Work out the finished part from the listing and answer in its coordinate system (mm). A direction names the side the tool comes from. Round coordinates to 2 decimals unless told otherwise and drop trailing zeros. Order: outer loops, then holes, each group sorted by start corner. A loop starts at its lowest first (then second) coordinate and runs counter-clockwise, first axis right, second up. Notation, with made-up numbers: (27.5, 14) -> (38.5, 14) arc R26 cw to (38.5, 39) -> close; hole circle Ø9 at (33.5, 19). An arc over 180 degrees is marked (long way). Use a Markdown table: item, result. Add a question column.
Item 1: A cutting plane is placed at C-C, the plane y = 7. Determine the outline of the cut face in (x, z).
Item 2: A cutting plane is placed at B-B, the plane z = -42.25. Determine the outline of the cut face in (x, y).
Item 3: A tool of negligible diameter and unlimited length cuts with its end or side. For faces 4 (the flat face through (35.5, -5, -46)), 5 (the flat face through (64, 0, -59)), 6 (the flat face through (48.733, 0, -46)), 7 (the flat face through (58, 0, -32)), from which of +Z, -Z, +X, -X, +Y, -Y can it reach the whole face along a straight path? Write none if from no direction.
Item 4: A cutting plane is placed at D-D, the plane x = 69. Determine the outline of the cut face in (y, z), plus the area to 3 significant figures.
Item 5: For a pull along Y with two mould halves and no side action, classify faces 1 (the flat face through (58, 0, -60)), 2 (the flat face through (34, -8, -46)), 3 (the flat face through (56, -10, -46)) as +Y half, -Y half, draft (parallel to the pull), parting line (faces both ways), or undercut.
Item 6: A cutting plane is placed at A-A, the plane y = 0. Determine the outline of the cut face in (x, z), plus the area to 3 significant figures.
Item 7: Flat-ended cylindrical pins translate along their axes: P1, Ø1.5, axis at y = 6, z = -44.5, coming from the +X side; P2, Ø5, axis at y = -3, z = -40, coming from the +X side; P3, Ø8, axis at x = 63.5, z = -46.5, coming from the -Y side. Find the tip coordinate at first contact, or state that the pin passes through.
Item 8: Find the intervals of material crossed by L1, parallel to X at y = 8.5, z = -42; L2, parallel to X at y = 1, z = -57.5; L3, parallel to X at y = -5.5, z = -52, in increasing order. Write a range as [from, to].
from build123d import *

# Parameters (mm, degrees)
PAD006_DEPTH            = 28
SKETCH015_W             = 8
SKETCH015_H             = 3
SKETCH015_W_2           = 15
SKETCH015_H_2           = 6
POCKET006_DEPTH         = 28.001
SKETCH016_W             = 20
SKETCH016_H             = 2.5
SKETCH016_W_2           = 18
SKETCH016_H_2           = 3
POCKET007_DEPTH         = 27.001
BODY005_PLACEMENT_ANGLE = 90


with BuildPart() as part:
    # Sketch014 → Pad006 (new body)
    with BuildSketch(Plane.XY):
        with BuildLine():
            Line((-3, -3), (-8, -3))
            Line((-8, -3), (-8, 0))
            Line((-8, 0), (8, 0))
            Line((8, 0), (8, -3))
            Line((8, -3), (3, -3))
            Line((3, -3), (3, -8))
            ThreePointArc((-3, -8), (0, -41.733201), (3, -8))
            Line((-3, -3), (-3, -8))
        make_face()
    extrude(amount=PAD006_DEPTH)

    # Sketch015 (on Face9 of Pad006) → Pocket006 (cut, through all)
    with BuildSketch(Plane(origin=(0, 0, 0), x_dir=(1, 0, 0), z_dir=(0, 0, -1))):
        with Locations((0, 29.733201)):
            Rectangle(SKETCH015_W, SKETCH015_H)
        with Locations((0, 19.233201)):
            Rectangle(SKETCH015_W_2, SKETCH015_H_2)
    extrude(amount=-POCKET006_DEPTH, mode=Mode.SUBTRACT)

    # Sketch016 (on Face4 of Pocket006) → Pocket007 (cut, through all)
    with BuildSketch(Plane(origin=(0, 0, 1), x_dir=(1, 0, 0), z_dir=(0, 0, -1))):
        with Locations((0, 23.483201)):
            Rectangle(SKETCH016_W, SKETCH016_H)
        with Locations((0, 30.933201)):
            Rectangle(SKETCH016_W_2, SKETCH016_H_2)
    extrude(amount=-POCKET007_DEPTH, mode=Mode.SUBTRACT)


with BuildPart() as part_1:
    # Body005 placement: moved
    add(part.part.moved(Location((32.5, 0, -60))).rotate(Axis((32.5, 0, -60), (0, 0, 1)), BODY005_PLACEMENT_ANGLE))


solid = part_1.part
Reported:
| question | item | result |
|---|---|---|
| 1 | outline | (32.5, -60) -> (35.5, -60) -> (35.5, -32) -> (32.5, -32) -> close; (41.74, -60) -> (48.73, -60) -> (48.73, -32) -> (41.74, -32) -> close; (54.73, -60) -> (72.73, -60) -> (72.73, -32) -> (64.93, -32) -> (64.93, -59) -> (61.93, -59) -> (61.93, -32) -> (57.23, -32) -> (57.23, -59) -> (54.73, -59) -> close |
| 2 | outline | (32.5, -8) -> (35.5, -8) -> (35.5, -3) -> (40.5, -3) arc R17 ccw (long way) to (40.5, 3) -> (35.5, 3) -> (35.5, 8) -> (32.5, 8) -> close; hole (48.73, -7.5) -> (54.73, -7.5) -> (54.73, -10) -> (57.23, -10) -> (57.23, 10) -> (54.73, 10) -> (54.73, 7.5) -> (48.73, 7.5) -> close; hole (60.73, -4) -> (61.93, -4) -> (61.93, -9) -> (64.93, -9) -> (64.93, 9) -> (61.93, 9) -> (61.93, 4) -> (60.73, 4) -> close |
| 3 | face 4 | +Z, -Z, -Y |
| 3 | face 5 | +Z |
| 3 | face 6 | +Z, -Z |
| 3 | face 7 | +Z, +X, -X, +Y, -Y |
| 4 | outline | (-12.27, -60) -> (12.27, -60) -> (12.27, -32) -> (-12.27, -32) -> close |
| 4 | area | 687 mm² |
| 5 | face 1 | draft |
| 5 | face 2 | -Y half |
| 5 | face 3 | undercut |
| 6 | outline | (32.5, -60) -> (48.73, -60) -> (48.73, -32) -> (32.5, -32) -> close; (54.73, -60) -> (60.73, -60) -> (60.73, -32) -> (57.23, -32) -> (57.23, -59) -> (54.73, -59) -> close; (63.73, -60) -> (74.23, -60) -> (74.23, -32) -> (64.93, -32) -> (64.93, -59) -> (63.73, -59) -> close |
| 6 | area | 817 mm² |
| 7 | P1 | x = 73.4 |
| 7 | P2 | x = 74.23 |
| 7 | P3 | y = -16.85 |
| 8 | L1 | [42.51, 54.73], [57.23, 61.93], [64.93, 71.96] |
| 8 | L2 | [32.5, 48.73], [57.23, 60.73], [64.93, 74.2] |
| 8 | L3 | [32.5, 35.5], [41.15, 48.73], [57.23, 61.93], [64.93, 73.32] |
